Source: CAD feature listing. Evaluate the final solid. Frame: model axes, mm. A direction names the side the tool comes from. Round coordinates to 2 decimals unless told otherwise and drop trailing zeros. Loops run counter-clockwise (first coordinate to the right, second up) from the corner with the lowest first, then second, coordinate; pieces in that order, holes last. Notation, with made-up numbers: (45, -36.75) -> (49, -36.75) arc R32 ccw to (49, -10.75) -> close; hole circle Ø10 at (76.5, 71.25). An arc over 180 degrees is marked (long way). Put each result on its own line as item: value. Start each with the question number.
1. Draft query along Z for faces 1 (the flat face through (33.5, -14, 0)), 2 (the cylindrical face through (43.08, 0.32, 9.44)), 3 (the cylindrical face through (43.08, 28.94, -0.05)). Return one class per face: pulls with the +Z half, pulls with the -Z half, needs draft (parallel to the pull), parting line crosses it, or undercut.
2. Cut plane B-B (y = 11.5). Return the cut outline in (x, z), then the cut area to 3 significant figures.
3. Contact query for flat-ended pins moving along their axis: pin 1 (8 mm diameter, centred on x = 25, z = 9, fed in from +Y); pin 2 (2 mm diameter, centred on x = -24, z = -7, fed in from +Y); pin 3 (3 mm diameter, centred on x = -14.5, z = -6, fed in from -Y). Output: stop coordinate, or through.
4. Cut plane D-D (y = -19). Return the cut outline in (x, z).
5. Cut plane A-A (z = -1). Return the cut outline in (x, y).
6. Set-up query: faces 4 (the flat face through (40, -7, 0)), 5 (the flat face through (-1, -31.5, 0)). Return all of +Z, -Z, +X, -X, +Y, -Y with unobstructed straight access to the full face (end or side cutting, diameter ignored); none if empty.
7. Material intervals for L1, parallel to X at y = -16.5, z = -0.75; L2, parallel to Y at x = 42, z = 2.5; L3, parallel to Z at x = -1.5, y = -23.5, sorted ascending.
8. Cut plane C-C (x = -21.5). Return the cut outline in (y, z), then the cut area to 3 significant figures.
```python
from build123d import *

# Parameters (mm, degrees)
BOSS_EXTRUDE1_DEPTH      = 12
BOSS_EXTRUDE1_DEPTH_BACK = 12
SKETCH1_W                = 91
SKETCH1_H                = 63
FILLET1_R                = 8.5
FILLET2_R                = 8.5
SKETCH2_W                = 7
SKETCH2_H                = 14
CUT_EXTRUDE1_DEPTH       = 12


with BuildPart() as part:
    # Sketch1 → Boss-Extrude1 (new, two sides: drawn at the far end of the back side and taken through both)
    with BuildSketch(Plane.XY.offset(-BOSS_EXTRUDE1_DEPTH_BACK)):
        Rectangle(SKETCH1_W, SKETCH1_H)
    extrude(amount=BOSS_EXTRUDE1_DEPTH + BOSS_EXTRUDE1_DEPTH_BACK)

    # Fillet1
    fillet1_edges = [part.edges().sort_by_distance(p)[0] for p in [
        (45.5, 0, 12),
        (-45.5, 0, -12),
        (0, 31.5, 12),
        (-45.5, 0, 12),
        (0, -31.5, 12),
        (0, -31.5, -12),
        (45.5, 0, -12),
        (0, 31.5, -12),
    ]]
    fillet(fillet1_edges, radius=FILLET1_R)

    # Fillet2
    # the kernel refuses this fillet: 8.5 mm, written as the material it takes off along each edge
    with BuildSketch(Plane(origin=(37, -23, -3.5), x_dir=(1, 0, 0), z_dir=(0, -1, 0))) as fillet2_piece_1_section:
        Polygon((0, 0), (FILLET2_R, 0), (FILLET2_R, -FILLET2_R), (0, -FILLET2_R), align=None)
    fillet2_piece_1 = extrude(amount=FILLET2_R, mode=Mode.PRIVATE)
    fillet2_piece_1 = fillet2_piece_1 - Plane(origin=(37, -23, -3.5), x_dir=(-0.7071067811865475, 0, 0.7071067811865475), z_dir=(0, -1, 0)) * Sphere(FILLET2_R, mode=Mode.PRIVATE)
    add(fillet2_piece_1, mode=Mode.SUBTRACT)
    with BuildSketch(Plane(origin=(-37, -23, -3.5), x_dir=(-1, 0, 0), z_dir=(0, -1, 0))) as fillet2_piece_2_section:
        Polygon((0, 0), (FILLET2_R, 0), (FILLET2_R, FILLET2_R), (0, FILLET2_R), align=None)
    fillet2_piece_2 = extrude(amount=FILLET2_R, mode=Mode.PRIVATE)
    fillet2_piece_2 = fillet2_piece_2 - Plane(origin=(-37, -23, -3.5), x_dir=(0.7071067811865475, 0, 0.7071067811865475), z_dir=(0, -1, 0)) * Sphere(FILLET2_R, mode=Mode.PRIVATE)
    add(fillet2_piece_2, mode=Mode.SUBTRACT)
    with BuildSketch(Plane(origin=(37, 23, -3.5), x_dir=(0, 1, 0), z_dir=(1, 0, 0))) as fillet2_piece_3_section:
        Polygon((0, 0), (FILLET2_R, 0), (FILLET2_R, -FILLET2_R), (0, -FILLET2_R), align=None)
    fillet2_piece_3 = extrude(amount=FILLET2_R, mode=Mode.PRIVATE)
    fillet2_piece_3 = fillet2_piece_3 - Plane(origin=(37, 23, -3.5), x_dir=(0, -0.7071067811865475, 0.7071067811865475), z_dir=(1, 0, 0)) * Sphere(FILLET2_R, mode=Mode.PRIVATE)
    add(fillet2_piece_3, mode=Mode.SUBTRACT)
    with BuildSketch(Plane(origin=(-37, 23, -3.5), x_dir=(0, 1, 0), z_dir=(-1, 0, 0))) as fillet2_piece_4_section:
        Polygon((0, 0), (FILLET2_R, 0), (FILLET2_R, FILLET2_R), (0, FILLET2_R), align=None)
    fillet2_piece_4 = extrude(amount=FILLET2_R, mode=Mode.PRIVATE)
    fillet2_piece_4 = fillet2_piece_4 - Plane(origin=(-37, 23, -3.5), x_dir=(0, -0.7071067811865475, 0.7071067811865475), z_dir=(-1, 0, 0)) * Sphere(FILLET2_R, mode=Mode.PRIVATE)
    add(fillet2_piece_4, mode=Mode.SUBTRACT)
    with BuildSketch(Plane(origin=(-37, 23, 3.5), x_dir=(0, 1, 0), z_dir=(-1, 0, 0))) as fillet2_piece_5_section:
        Polygon((0, 0), (FILLET2_R, 0), (FILLET2_R, -FILLET2_R), (0, -FILLET2_R), align=None)
    fillet2_piece_5 = extrude(amount=FILLET2_R, mode=Mode.PRIVATE)
    fillet2_piece_5 = fillet2_piece_5 - Plane(origin=(-37, 23, 3.5), x_dir=(0, -0.7071067811865475, -0.7071067811865475), z_dir=(-1, 0, 0)) * Sphere(FILLET2_R, mode=Mode.PRIVATE)
    add(fillet2_piece_5, mode=Mode.SUBTRACT)
    with BuildSketch(Plane(origin=(37, 23, 3.5), x_dir=(0, 1, 0), z_dir=(1, 0, 0))) as fillet2_piece_6_section:
        Polygon((0, 0), (FILLET2_R, 0), (FILLET2_R, FILLET2_R), (0, FILLET2_R), align=None)
    fillet2_piece_6 = extrude(amount=FILLET2_R, mode=Mode.PRIVATE)
    fillet2_piece_6 = fillet2_piece_6 - Plane(origin=(37, 23, 3.5), x_dir=(0, -0.7071067811865475, -0.7071067811865475), z_dir=(1, 0, 0)) * Sphere(FILLET2_R, mode=Mode.PRIVATE)
    add(fillet2_piece_6, mode=Mode.SUBTRACT)
    with BuildSketch(Plane(origin=(-37, -23, 3.5), x_dir=(-1, 0, 0), z_dir=(0, -1, 0))) as fillet2_piece_7_section:
        Polygon((0, 0), (FILLET2_R, 0), (FILLET2_R, -FILLET2_R), (0, -FILLET2_R), align=None)
    fillet2_piece_7 = extrude(amount=FILLET2_R, mode=Mode.PRIVATE)
    fillet2_piece_7 = fillet2_piece_7 - Plane(origin=(-37, -23, 3.5), x_dir=(0.7071067811865475, 0, -0.7071067811865475), z_dir=(0, -1, 0)) * Sphere(FILLET2_R, mode=Mode.PRIVATE)
    add(fillet2_piece_7, mode=Mode.SUBTRACT)
    with BuildSketch(Plane(origin=(37, -23, 3.5), x_dir=(1, 0, 0), z_dir=(0, -1, 0))) as fillet2_piece_8_section:
        Polygon((0, 0), (FILLET2_R, 0), (FILLET2_R, FILLET2_R), (0, FILLET2_R), align=None)
    fillet2_piece_8 = extrude(amount=FILLET2_R, mode=Mode.PRIVATE)
    fillet2_piece_8 = fillet2_piece_8 - Plane(origin=(37, -23, 3.5), x_dir=(-0.7071067811865475, 0, -0.7071067811865475), z_dir=(0, -1, 0)) * Sphere(FILLET2_R, mode=Mode.PRIVATE)
    add(fillet2_piece_8, mode=Mode.SUBTRACT)
    with BuildSketch(Plane(origin=(-45.5, 31.5, 3.5), x_dir=(0, -1, 0), z_dir=(0, 0, -1)), Plane(origin=(45.5, 31.5, -3.5), x_dir=(0, -1, 0), z_dir=(0, 0, 1)), Plane(origin=(-45.5, -31.5, 3.5), x_dir=(1, 0, 0), z_dir=(0, 0, -1)), Plane(origin=(45.5, -31.5, -3.5), x_dir=(-1, 0, 0), z_dir=(0, 0, 1))) as fillet2_piece_9:
        with BuildLine():
            CenterArc((FILLET2_R, -FILLET2_R), FILLET2_R, 90, 90)
            Line((0, -FILLET2_R), (0, 0))
            Line((0, 0), (FILLET2_R, 0))
        make_face()
    extrude(amount=7, mode=Mode.SUBTRACT)

    # Sketch2 → Cut-Extrude1 (cut)
    with BuildSketch(Plane(origin=(45.5, 0, 0), x_dir=(0, 0, -1), z_dir=(1, 0, 0))):
        with Locations((0, -14)):
            Rectangle(SKETCH2_W, SKETCH2_H)
    extrude(amount=-CUT_EXTRUDE1_DEPTH, mode=Mode.SUBTRACT)


solid = part.part
```
Solution:
1. face 1: undercut
1. face 2: pulls with the +Z half
1. face 3: needs draft
2. outline: (-45.5, -3.5) arc R8.5 ccw to (-37, -12) -> (37, -12) arc R8.5 ccw to (45.5, -3.5) -> (45.5, 3.5) arc R8.5 ccw to (37, 12) -> (-37, 12) arc R8.5 ccw to (-45.5, 3.5) -> close
2. area: 2,120 mm^2
3. pin 1: stops at y = 31.37
3. pin 2: stops at y = 31.12
3. pin 3: stops at y = -31.44
4. outline: (-45.5, -3.5) arc R8.5 ccw to (-37, -12) -> (37, -12) arc R8.5 ccw to (45.5, -3.5) -> (33.5, -3.5) -> (33.5, 3.5) -> (45.5, 3.5) arc R8.5 ccw to (37, 12) -> (-37, 12) arc R8.5 ccw to (-45.5, 3.5) -> close
5. outline: (-45.5, -23) arc R8.5 ccw to (-37, -31.5) -> (37, -31.5) arc R8.5 ccw to (45.5, -23) -> (45.5, -21) -> (33.5, -21) -> (33.5, -7) -> (45.5, -7) -> (45.5, 23) arc R8.5 ccw to (37, 31.5) -> (-37, 31.5) arc R8.5 ccw to (-45.5, 23) -> close
6. face 4: +X
6. face 5: +Z, -Z, +X, -X, -Y
7. L1: x = -45.5 to 33.5
7. L2: y = -29.87 to -21, -7 to 29.87
7. L3: z = -11.99 to 11.99
8. outline: (-31.5, -3.5) arc R8.5 ccw to (-23, -12) -> (23, -12) arc R8.5 ccw to (31.5, -3.5) -> (31.5, 3.5) arc R8.5 ccw to (23, 12) -> (-23, 12) arc R8.5 ccw to (-31.5, 3.5) -> close
8. area: 1,450 mm^2
